Geometry: see drawing. Coordinates: mm, zero at the bounding-box minimum. Give positions to 0.01 mm unless a question says otherwise; leave off trailing zeros. Loops run counter-clockwise (first coordinate to the right, second up) from the corner with the lowest first, then second, coordinate; pieces in that order, holes last. Notation, with made-up numbers: M -38,-6 L -30,-6 A21 ccw -30,17 Z; hole C -28.5,27 d4. An arc over 180 degrees is marked long. Put each result on its own line as item: value.
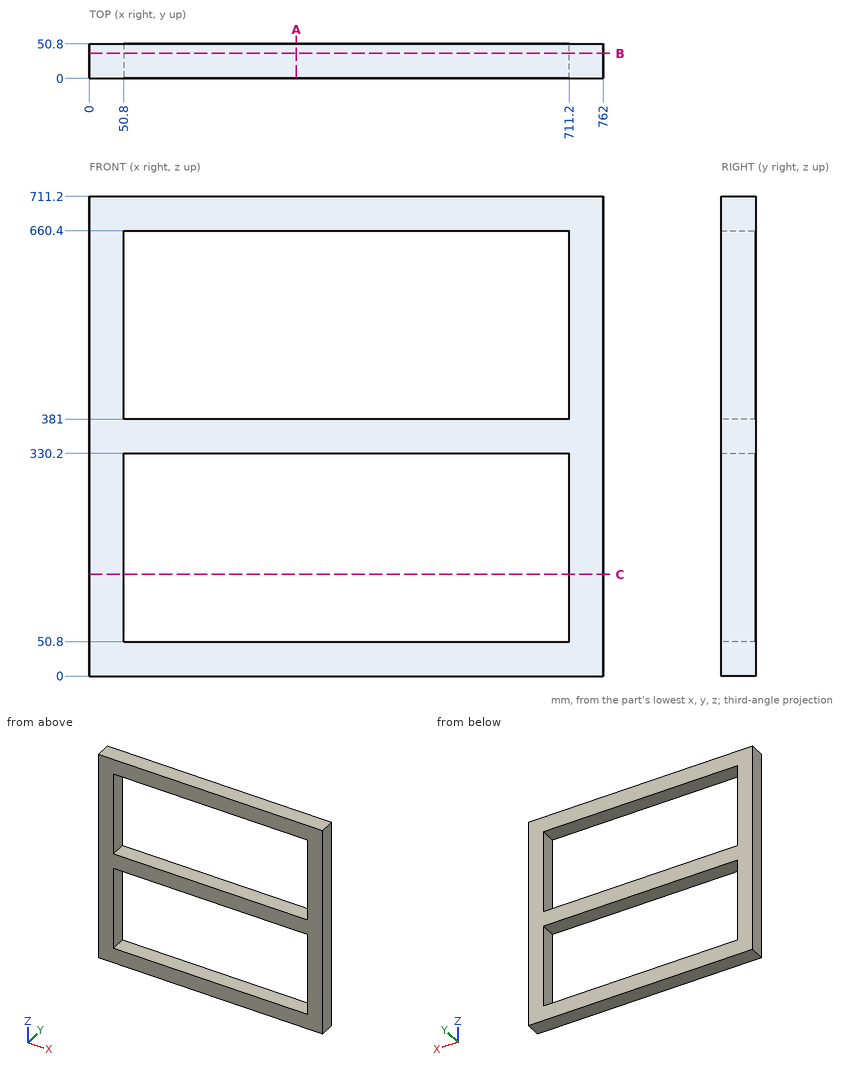
1. Material intervals for line 1 (Z direction, x = 393.5, y = 43.5); line 2 (X direction, y = 36.5, z = 196.5), sorted ascending. Write a range as from..to.
Found:
line 1: 0..50.8, 330.2..381, 660.4..711.2
line 2: 0..50.8, 711.2..762
2. Section query B-B (y = 37). Output: boundary loops of the cut face in (x, z).
Found:
outline: M 0,0 L 762,0 L 762,711.2 L 0,711.2 Z; hole M 50.8,50.8 L 711.2,50.8 L 711.2,330.2 L 50.8,330.2 Z; hole M 50.8,381 L 711.2,381 L 711.2,660.4 L 50.8,660.4 Z
3. Section query A-A (x = 307). Output: boundary loops of the cut face in (y, z), plus the area to 3 significant figures.
Found:
outline: M 0,0 L 50.8,0 L 50.8,50.8 L 0,50.8 Z; M 0,330.2 L 50.8,330.2 L 50.8,381 L 0,381 Z; M 0,660.4 L 50.8,660.4 L 50.8,711.2 L 0,711.2 Z
area: 7,740 mm^2
4. Section query C-C (z = 150.5). Output: boundary loops of the cut face in (x, y).
Found:
outline: M 0,0 L 50.8,0 L 50.8,50.8 L 0,50.8 Z; M 711.2,0 L 762,0 L 762,50.8 L 711.2,50.8 Z
5. Contact query for a flat-ended pin moving along its axis: P1, Ø15, axis at y = 19.5, z = 466.5, coming from the -X side. Output: stop coordinate, or through.
Found:
P1: x = 0
